The figure shows three views and two pictorial views of one solid part (mm, origin at its lowest corner). Answer the questions. A direction names the side the tool comes from. Coordinates: 2 decimals unless noted, no trailing zeros. Write each loop counter-clockwise with the first axis right and the second up, starting at its lowest first coordinate (ties: lowest second). Pieces come first, ordered by that corner, then holes. Notation, with made-up numbers: M 37,54.25 L 68,54.25 A19 cw 68,72.25 Z; hole C 37,-1.5 d3. An arc over 180 degrees is marked long. Answer as CSV lines item,"result".
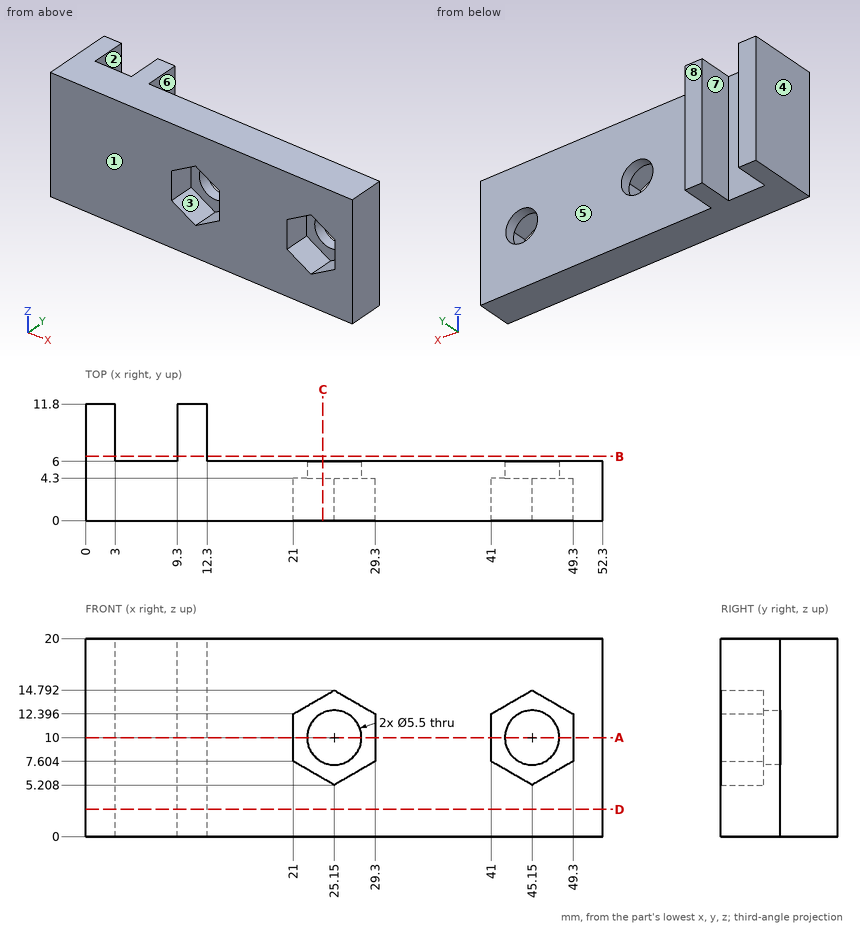
Q1. Straight lines are drawn through the part: line 1 (X direction, y = 0.5, z = 10.25); line 2 (X direction, y = 5.6, z = 10); line 3 (Z direction, x = 45.15, y = 5.3). For each, find the intervals that lie inside material, in ascending order.
Output:
line 1,"0 to 21, 29.3 to 41, 49.3 to 52.3"
line 2,"0 to 22.4, 27.9 to 42.4, 47.9 to 52.3"
line 3,"0 to 7.25, 12.75 to 20"
Q2. Find section D-D (z = 2.75). Give the vertices of the cut face in (x, y).
Output:
outline,"M 0,0 L 52.3,0 L 52.3,6 L 12.3,6 L 12.3,11.8 L 9.3,11.8 L 9.3,6 L 3,6 L 3,11.8 L 0,11.8 Z"
Q3. Flat-ended cylindrical pins translate along their axes: pin 1 Ø6 at (x, z) = (40, 8) entering from +Y; pin 2 Ø6.5 at (y, z) = (9.5, 8) entering from +X. Find the tip coordinate at first contact, or state that the pin passes through.
Output:
pin 1,"y = 6"
pin 2,"x = 12.3"
Q4. Find section C-C (x = 24). Give the vertices of the cut face in (y, z).
Output:
outline,"M 0,0 L 6,0 L 6,7.5 L 4.3,7.5 L 4.3,5.87 L 0,5.87 Z; M 0,14.13 L 4.3,14.13 L 4.3,12.5 L 6,12.5 L 6,20 L 0,20 Z"
Q5. Find section B-B (y = 6.5). Give the vertices of the cut face in (x, z).
Output:
outline,"M 0,0 L 3,0 L 3,20 L 0,20 Z; M 9.3,0 L 12.3,0 L 12.3,20 L 9.3,20 Z"
Q6. Find section A-A (z = 10). Give the vertices of the cut face in (x, y).
Output:
outline,"M 0,0 L 21,0 L 21,4.3 L 22.4,4.3 L 22.4,6 L 12.3,6 L 12.3,11.8 L 9.3,11.8 L 9.3,6 L 3,6 L 3,11.8 L 0,11.8 Z; M 27.9,4.3 L 29.3,4.3 L 29.3,0 L 41,0 L 41,4.3 L 42.4,4.3 L 42.4,6 L 27.9,6 Z; M 47.9,4.3 L 49.3,4.3 L 49.3,0 L 52.3,0 L 52.3,6 L 47.9,6 Z"
Q7. For the marked faces 1, 2, 3, 4 and 5, determine the directions among +Z, -Z, +X, -X, +Y, -Y from which every point of the face is accessible in a straight line to the end or side of a thin tool.
Output:
face 1,"+Z, -Z, +X, -X, -Y"
face 2,"+Z, -Z, +Y"
face 3,"-Y"
face 4,"+Z, -Z, -X, +Y, -Y"
face 5,"+Z, -Z, +X, +Y"
Q8. The mould has two halves that part along X. Classify the marked faces 6, 7 and 8: pulls with the +X half, pulls with the -X half, needs draft (parallel to the pull), parting line crosses it, or undercut.
Output:
face 6,"pulls with the +X half"
face 7,"undercut"
face 8,"needs draft"
